Can you work these out from the model? Positions are in its coordinate system, mm. A direction names the side the tool comes from. Give positions to 0.01 mm unless a question says otherwise; leave off trailing zeros. Write each loop counter-clockwise with the first axis right and the second up, starting at its lowest first coordinate (ties: lowest second). Pieces come first, ordered by that corner, then holes.
1. Suppose I cut it at A-A (z = 84.5). Please give me the cut outline in (x, y).
2. Thinking about a two-plate mould opening in Z: for faces 1 (the cylindrical face through (-1.613, 6.892, 123.844)), 2 (the flat face through (0, -6.3, 99)), 3 (the flat face through (-7, 0, 0)), which applies, pulls with the +Z half, pulls with the -Z half, needs draft (parallel to the pull), parting line crosses it, or undercut?
3. On a 3-axis mill with a long thin cutter (end or side, diameter ignored), from which of +Z, -Z, +X, -X, +Y, -Y can I reach the whole of each face in a straight line? I mean faces 4 (the cylindrical face through (-1.613, 6.892, 133.844)), 5 (the flat face through (-6.3, 0, 99)). Say none if no direction works.
4. I'm going to push flat-ended pins straight in: pin 1 (1.9 mm diameter, centred on x = -1, z = 125.32, fed in from -Y); pin 2 (4 mm diameter, centred on x = -6, y = 0, fed in from +Z). Where does each tip first touch, or does it pass through?
5. If I drill on probe 1 along Y at (x, z) = (-0.5, 10), over which ranges is the centre line in solid material (lowest first)?
6. Suppose I cut it at B-B (y = 3.5). Please give me the cut outline in (x, z).
```python
from build123d import *

# Parameters (mm, degrees)
SKETCH_1_W          = 15
SKETCH_1_H          = 15
SKETCH_1_W_2        = 12.6
SKETCH_1_H_2        = 12.6
EXTRUDE_1_DEPTH     = 200
SKETCH_2_R          = 1.6
CUT_EXTRUDE_1_DEPTH = 25


with BuildPart() as part:
    # 草图1 → 凸台-拉伸1 (new body)
    with BuildSketch(Plane.XY):
        Rectangle(SKETCH_1_W, SKETCH_1_H)
        Rectangle(SKETCH_1_W_2, SKETCH_1_H_2, mode=Mode.SUBTRACT)
    extrude(amount=EXTRUDE_1_DEPTH)

    # 草图2 → 切除-拉伸1 (cut)
    with BuildSketch(Plane.XZ.offset(7.5)):
        with Locations(Location((-1, 135.322387076, 0), (0, 0, 270))):
            Circle(SKETCH_2_R)
        with Locations(Location((-1, 125.322387076, 0), (0, 0, 270))):
            Circle(SKETCH_2_R)
    extrude(amount=-CUT_EXTRUDE_1_DEPTH, mode=Mode.SUBTRACT)


solid = part.part
```
Checks:
1. outline: (-7.5, -7.5) - (7.5, -7.5) - (7.5, 7.5) - (-7.5, 7.5) - close; hole (-6.3, -6.3) - (6.3, -6.3) - (6.3, 6.3) - (-6.3, 6.3) - close
2. face 1: undercut
2. face 2: needs draft
2. face 3: pulls with the -Z half
3. face 4: +Y, -Y
3. face 5: +Z, -Z
4. pin 1: passes through
4. pin 2: stops at z = 200
5. probe 1: y = -7.5 to -6.3, 6.3 to 7.5
6. outline: (-7.5, 0) - (-6.3, 0) - (-6.3, 200) - (-7.5, 200) - close; (6.3, 0) - (7.5, 0) - (7.5, 200) - (6.3, 200) - close
